from build123d import *

# Parameters (mm, degrees)
BOSS_EXTRUDE4_REACH = 79.782
SKETCH4_R           = 25
SKETCH5_R           = 24
CUT_EXTRUDE5_DEPTH  = 15


with BuildPart() as part:
    # Sketch1 → Revolve1 (revolve)
    with BuildSketch(Plane(origin=(0, 0, 0), x_dir=(0, 0, -1), z_dir=(1, 0, 0)), mode=Mode.PRIVATE) as revolve1_sk:
        Polygon((0, 0), (0, -10), (19, -10), (19, -7), (22, -7), (22, -10), (27, -10), (27, -7), (30, -7), (30, -10), (35, -10), (35, 25), (15, 25), (15, 0), align=None)
    revolve(revolve1_sk.sketch.rotate(Axis((0, 25, -35), (0, 0, 1)), 180), axis=Axis((0, 25, -35), (0, 0, 1)))

    # Sketch4 → Boss-Extrude4 (add, up to next)
    with BuildSketch(Plane.XY, mode=Mode.PRIVATE) as boss_extrude4_sk1:
        with Locations((0, 25)):
            Circle(SKETCH4_R)
    boss_extrude4_tool1 = extrude(boss_extrude4_sk1.sketch, amount=-BOSS_EXTRUDE4_REACH, mode=Mode.PRIVATE) - part.part
    add(boss_extrude4_tool1.solids().sort_by_distance((0, 25, 0))[0])

    # Sketch5 → Cut-Extrude5 (cut)
    with BuildSketch(Plane(origin=(0, 0, -35), x_dir=(-1, 0, 0), z_dir=(0, 0, -1))):
        with Locations(Location((0, 25, 0), (0, 0, 90))):
            Circle(SKETCH5_R)
    extrude(amount=-CUT_EXTRUDE5_DEPTH, mode=Mode.SUBTRACT)


solid = part.part
Geometry check sheet. Reference: the model listing, model coordinates, mm. A direction names the side the tool comes from. Round coordinates to 2 decimals unless told otherwise and drop trailing zeros. Order: outer loops, then holes, each group sorted by start corner. A loop starts at its lowest first (then second) coordinate and runs counter-clockwise, first axis right, second up. Notation, with made-up numbers: M 17.5,81.25 L 55.5,81.25 A25 ccw 55.5,119.25 Z; hole C 23,-5.5 d11. An arc over 180 degrees is marked long. Answer in a Markdown table with one row per item.
(1) Tool access check on faces 1 (the face through (1.055, 1.023, -27.605)), 2 (the face through (34.168, 17.413, -24.535)), 3 (the face through (15.4, -3.4, -30)). Record the directions out of +Z, -Z, +X, -X, +Y, -Y that give a thin tool (end or side, any length) a straight path to the whole face; none if there is none.
Responses:
| item | result |
|---|---|
| face 1 | -Z |
| face 2 | +Z, -Z |
| face 3 | none |
(2) Sectioned sample at A-A, the plane z = -26. Record the cut outline in (x, y), and give its area (3 significant figures).
Responses:
| item | result |
|---|---|
| outline | C 0,25 d70; hole C 0,25 d48 |
| area | 2,040 mm² |
(3) Scan lines: probe 1 along Z at (x, y) = (-27, 7); probe 2 along X at (y, z) = (25, -26.25); probe 3 along X at (y, z) = (25, -28). Record each from-to range of solid material in increasing order. Write a range as from..to.
Responses:
| item | result |
|---|---|
| probe 1 | z = -35..-30, -27..-22, -19..0 |
| probe 2 | x = -35..-24, 24..35 |
| probe 3 | x = -32..-24, 24..32 |
(4) Sectioned sample at D-D, the plane z = -15. Record the cut outline in (x, y).
Responses:
| item | result |
|---|---|
| outline | C 0,25 d70 |
(5) Sectioned sample at B-B, the plane x = 0. Record the cut outline in (y, z).
Responses:
| item | result |
|---|---|
| outline | M -10,-35 L 1,-35 L 1,-20 L 49,-20 L 49,-35 L 60,-35 L 60,-30 L 57,-30 L 57,-27 L 60,-27 L 60,-22 L 57,-22 L 57,-19 L 60,-19 L 60,0 L -10,0 L -10,-19 L -7,-19 L -7,-22 L -10,-22 L -10,-27 L -7,-27 L -7,-30 L -10,-30 Z |
(6) Sectioned sample at C-C, the plane y = 25. Record the cut outline in (x, z).
Responses:
| item | result |
|---|---|
| outline | M -35,-35 L -24,-35 L -24,-20 L 24,-20 L 24,-35 L 35,-35 L 35,-30 L 32,-30 L 32,-27 L 35,-27 L 35,-22 L 32,-22 L 32,-19 L 35,-19 L 35,0 L -35,0 L -35,-19 L -32,-19 L -32,-22 L -35,-22 L -35,-27 L -32,-27 L -32,-30 L -35,-30 Z |
(7) Draft check along Z on faces 4 (the face through (0, 25, 0)), 5 (the face through (0, 25, -20)), 6 (the face through (28.4, 40.4, -27)), 7 (the face through (34.168, 17.413, -9.633)). Enter one of: released by +Z, released by -Z, zero draft, split by the parting line, or undercut.
Responses:
| item | result |
|---|---|
| face 4 | released by +Z |
| face 5 | released by -Z |
| face 6 | undercut |
| face 7 | zero draft |
(8) Go/stop test with flat-tipped pins: P1, Ø21, axis at x = -4, y = 26.5, coming from the -Z side; P2, Ø12, axis at y = 39.5, z = -22.5, coming from the +X side; P3, Ø2, axis at y = 50.5, z = -7.5, coming from the -X side (3 decimals). Record where each tip stops, or that it passes through.
Responses:
| item | result |
|---|---|
| P1 | stops at z = -20 |
| P2 | stops at x = 33.95 |
| P3 | stops at x = -24.995 |
